Design review of the part shown in the three views and the two pictorial views. Dimensions are in mm from the part's minimum x, y and z. A direction names the side the tool comes from. Give positions to 0.01 mm unless a question says otherwise; leave off trailing zeros. Loops run counter-clockwise (first coordinate to the right, second up) from the corner with the lowest first, then second, coordinate; pieces in that order, holes last. Notation, with made-up numbers: (78, 79.25) - (120, 79.25) arc R16 ccw to (120, 88.25) - close; hole circle Ø8 at (84, -38.75). An arc over 180 degrees is marked (long way). Answer in a Markdown table with one row per item.
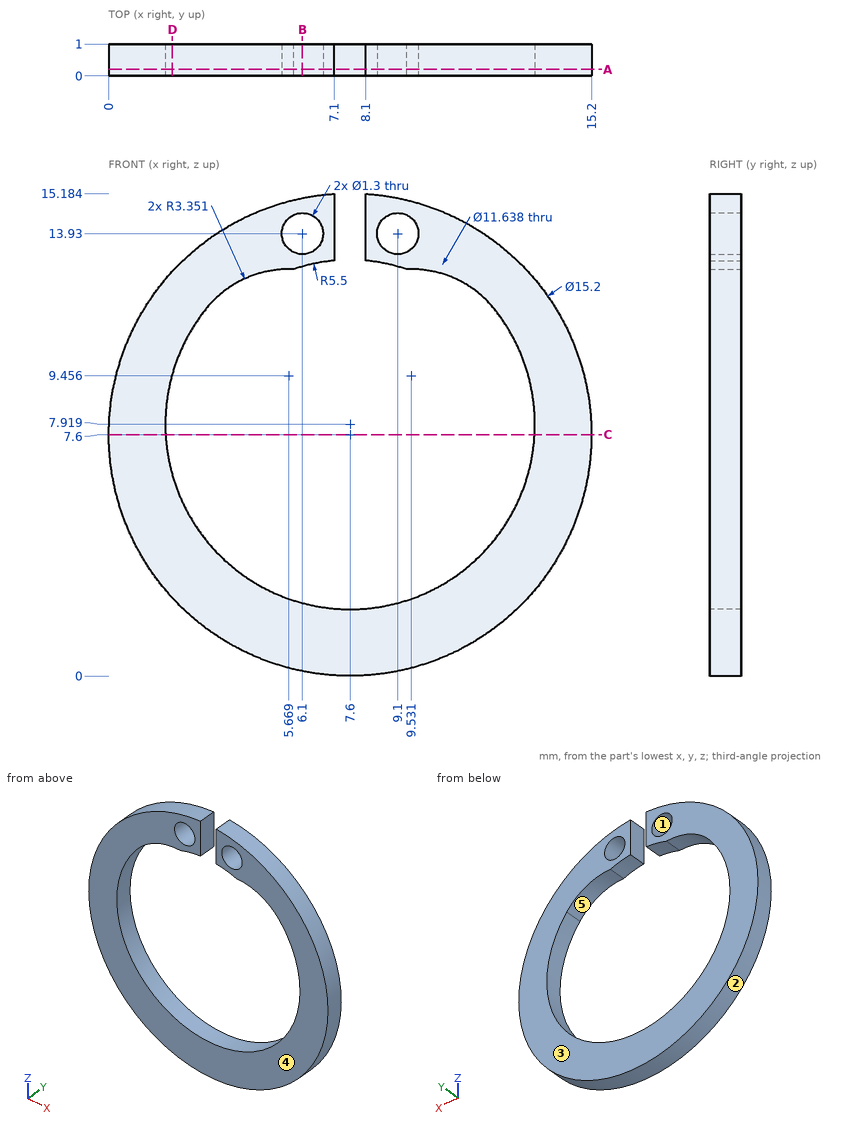
1. We need section B-B, the plane x = 6.1. Give the boundary of the cut face in (y, z).
Values:
| item | result |
|---|---|
| outline | (0, 0.15) - (1, 0.15) - (1, 2.3) - (0, 2.3) - close; (0, 12.89) - (1, 12.89) - (1, 13.28) - (0, 13.28) - close; (0, 14.58) - (1, 14.58) - (1, 15.05) - (0, 15.05) - close |
2. Mouldability with a two-part tool opening along X and no side actions: class the marked faces 1, 2 and 3 as released by +X, released by -X, zero draft, split by the parting line, or undercut.
Values:
| item | result |
|---|---|
| face 1 | undercut |
| face 2 | split by the parting line |
| face 3 | zero draft |
3. We need section A-A, the plane y = 0.2. Give the boundary of the cut face in (x, z).
Values:
| item | result |
|---|---|
| outline | (3.05, 11.54) arc R3.35 cw to (5.82, 12.8) arc R5.5 cw to (7.1, 13.08) - (7.1, 15.18) arc R7.6 ccw (long way) to (8.1, 15.18) - (8.1, 13.08) arc R5.5 cw to (9.38, 12.8) arc R3.35 cw to (12.15, 11.54) arc R5.82 cw (long way) to start; hole circle Ø1.3 at (6.1, 13.93); hole circle Ø1.3 at (9.1, 13.93) |
4. We need section D-D, the plane x = 2. Give the boundary of the cut face in (y, z).
Values:
| item | result |
|---|---|
| outline | (0, 2.46) - (1, 2.46) - (1, 6.34) - (0, 6.34) - close; (0, 9.5) - (1, 9.5) - (1, 12.74) - (0, 12.74) - close |
5. Wall thickness on line 1 (Z direction, x = 9.25, y = 0.7); line 2 (X direction, y = 0.2, z = 5.5) (1 decimal); line 3 (Z direction, x = 10.75, y = 0.2) (1 decimal): over which ranges is each line inside the solid? List them lowest first. Write a range as [from, to].
Values:
| item | result |
|---|---|
| line 1 | z = [0.18, 2.34], [12.85, 13.3], [14.56, 15.02] |
| line 2 | x = [0.3, 2.3], [12.9, 14.9] |
| line 3 | z = [0.7, 3], [12.6, 14.5] |
6. We need section C-C, the plane z = 7.6. Give the boundary of the cut face in (x, y).
Values:
| item | result |
|---|---|
| outline | (0, 0) - (1.79, 0) - (1.79, 1) - (0, 1) - close; (13.41, 0) - (15.2, 0) - (15.2, 1) - (13.41, 1) - close |
7. For the marked faces 4 and 5, list the 3-axis set-ups (+Z, -Z, +X, -X, +Y, -Y) from which the entire face can be reached by the end or side of a thin tool; tool diameter is ignored.
Values:
| item | result |
|---|---|
| face 4 | +Z, -Z, +X, -X, -Y |
| face 5 | +Y, -Y |
